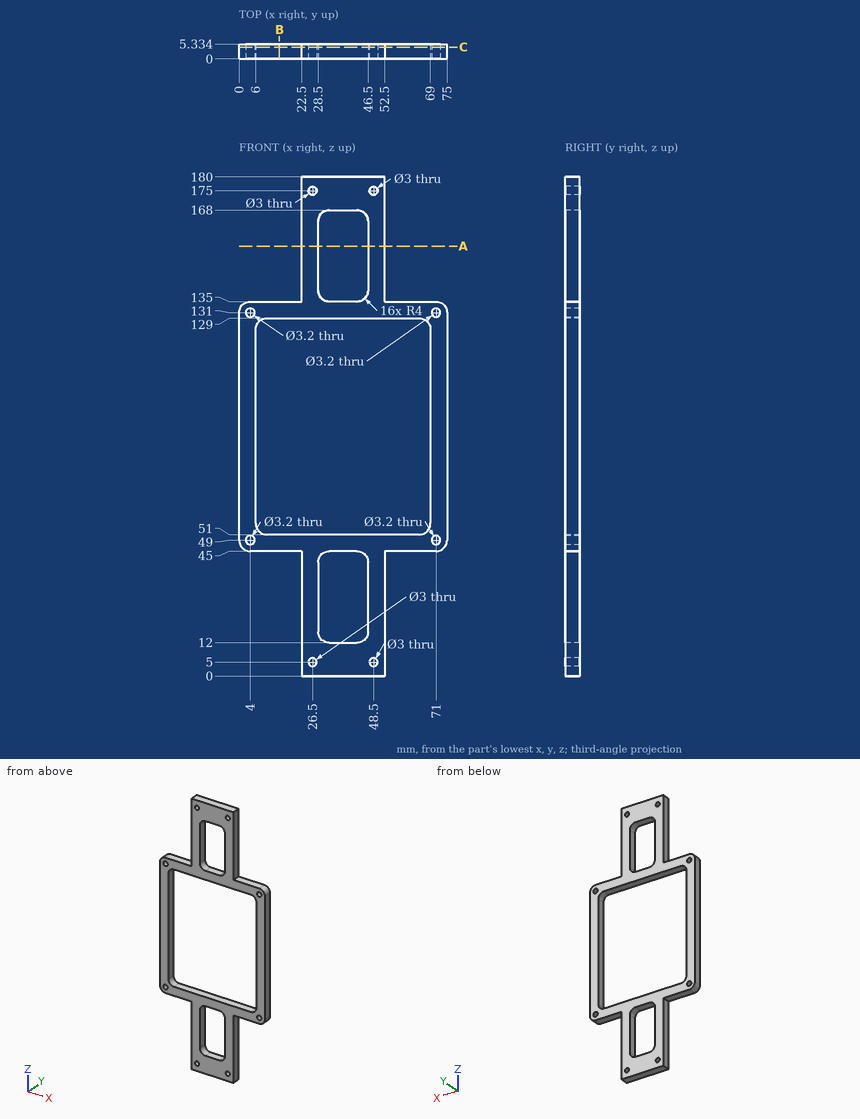
Here's the drawing with two shaded views (mm, measured from the low corner). I have some questions. Round coordinates to 2 decimals unless told otherwise and drop trailing zeros. Write each loop counter-clockwise with the first axis right and the second up, starting at its lowest first coordinate (ties: lowest second). Pieces come first, ordered by that corner, then holes. Notation, with made-up numbers: M -12.5,63.5 L 5.5,63.5 A5 cw 5.5,68.5 Z; hole C 18.25,44.5 d9. An arc over 180 degrees is marked long. Write each question's results on one line, items separated by ' | '. Start each with the question number.
1. Imagine slicing it at A-A on z = 155. List the corners of the cut face in (x, y) for me, and give its area (3 significant figures).
2. I need wall thicknesses on L1, parallel to X at y = 3.65, z = 49; L2, parallel to Z at x = 35, y = 3.2; L3, parallel to X at y = 3.05, z = 175. Which ranges of each line are inside material? Lowest first, please. Write a range as from..to.
3. Imagine slicing it at B-B on x = 14.5. List the corners of the cut face in (y, z) for me, and give its area (3 significant figures).
4. I'm going to push flat-ended pins straight in: pin 1 Ø2.5 at (x, z) = (48.5, 175) entering from +Y; pin 2 Ø2.5 at (y, z) = (4, 29.5) entering from +X; pin 3 Ø1.6 at (y, z) = (3.5, 21) entering from -X; pin 4 Ø1 at (x, y) = (67, 2) entering from +Z. Where does each tip first touch, or does it pass through?
5. Imagine slicing it at C-C on y = 4.2. Count the separate pieces of the cut face and the enclosed holes in it, and give its area (3 significant figures).
Result sheet:
1) outline: M 22.5,0 L 28.5,0 L 28.5,5.33 L 22.5,5.33 Z; M 46.5,0 L 52.5,0 L 52.5,5.33 L 46.5,5.33 Z | area: 64.0 mm^2
2) L1: x = 0..2.4, 5.6..69.4, 72.6..75 | L2: z = 0..12, 45..51, 129..135, 168..180 | L3: x = 22.5..25, 28..47, 50..52.5
3) outline: M 0,45 L 5.33,45 L 5.33,51 L 0,51 Z; M 0,129 L 5.33,129 L 5.33,135 L 0,135 Z | area: 64.0 mm^2
4) pin 1: passes through | pin 2: stops at x = 52.5 | pin 3: stops at x = 22.5 | pin 4: stops at z = 135
5) separate pieces: 1 | enclosed holes: 11 | area: 3,320 mm^2
